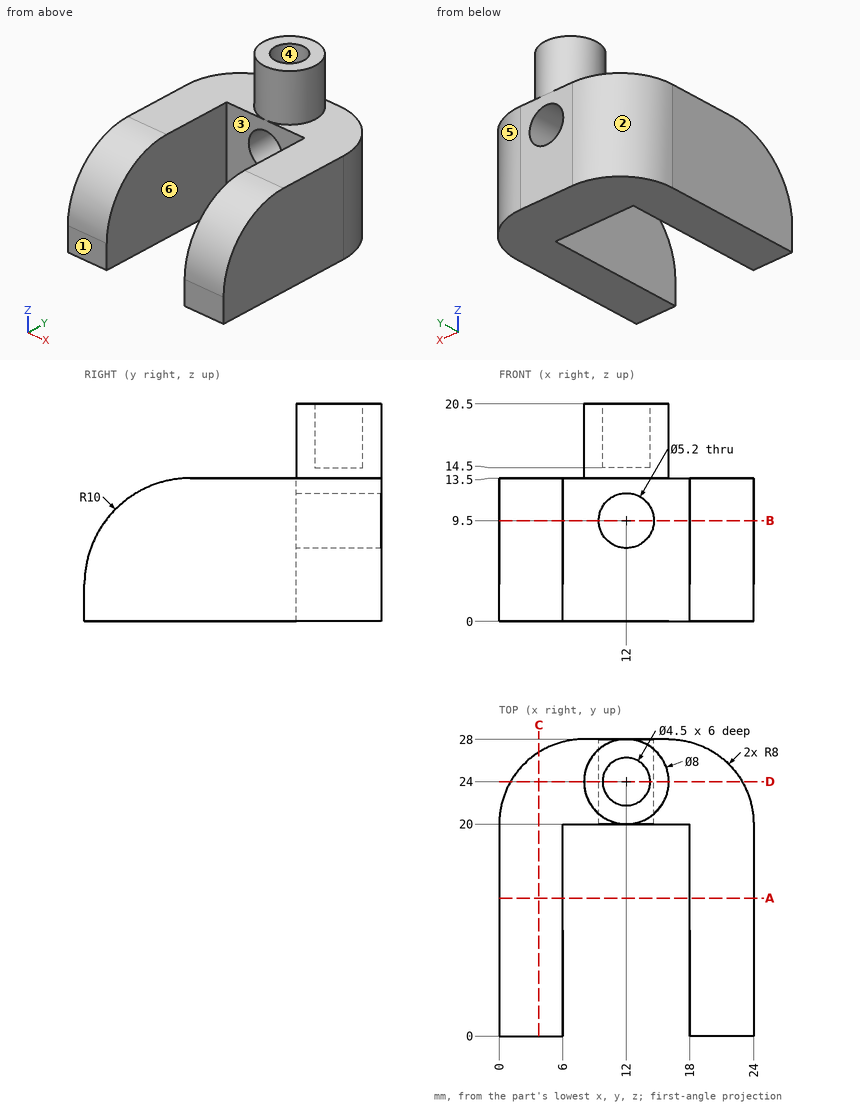
For this review, use the dimensioned drawing (mm, ordinates from the lowest corner) and the shaded views. A direction names the side the tool comes from. Give positions to 0.01 mm unless a question says otherwise; leave off trailing zeros. Order: outer loops, then holes, each group sorted by start corner. A loop starts at its lowest first (then second) coordinate and runs counter-clockwise, first axis right, second up. Notation, with made-up numbers: (37, -14) - (66, -14) arc R23 ccw to (66, -3) - close; hole circle Ø11 at (2, 6). An arc over 180 degrees is marked (long way). Use CSV: the item, a comma, the result in double quotes. Start each with the question number.
Q1. For line 1 (X direction, y = 24, z = 17); line 2 (X direction, y = 18.5, z = 2.75); line 3 (Z direction, x = 12, y = 25), list the stretches that pass through material, from the lowest coordinate up.
Q2. Take a section at A-A (y = 13). State the section outline as (x, z) points, and give its area (3 significant figures).
Q3. For P1, Ø4, axis at x = 12, y = 24, coming from the +Z side; P2, Ø1.5, axis at y = 24, z = 4.5, coming from the -X side; P3, Ø7, axis at x = 12, z = 9.5, coming from the -Y side, all flat-tipped, find the tip position at first contact; note any pin that passes through.
Q4. Draft analysis for pull direction X (two halves, no side actions). For the marked faces 1, 2 and 3, state which applies: pulls with the +X half, pulls with the -X half, needs draft (parallel to the pull), parting line crosses it, or undercut.
Q5. Take a section at D-D (y = 24). State the section outline as (x, z) points.
Q6. Take a section at B-B (z = 9.5). State the section outline as (x, y) points, and give its area (3 significant figures).
Q7. Machinability: for the marked faces 4, 5 and 6, which of the approach directions +Z, -Z, +X, -X, +Y, -Y give a long, thin tool a straight path to every point of the face, cutting with its end or side? Answer none if there is none.
Q8. Take a section at C-C (x = 3.75). State the section outline as (y, z) points.
Calculated:
1,line 1,"x = 8 to 9.75, 14.25 to 16"
1,line 2,"x = 0 to 6, 18 to 24"
1,line 3,"z = 0 to 6.9, 12.1 to 14.5"
2,outline,"(0, 0) - (6, 0) - (6, 13.5) - (0, 13.5) - close; (18, 0) - (24, 0) - (24, 13.5) - (18, 13.5) - close"
2,area,"162 mm²"
3,P1,"stops at z = 14.5"
3,P2,"stops at x = 0.69"
3,P3,"stops at y = 20"
4,face 1,"needs draft"
4,face 2,"pulls with the -X half"
4,face 3,"undercut"
5,outline,"(1.07, 0) - (22.93, 0) - (22.93, 13.5) - (16, 13.5) - (16, 20.5) - (14.25, 20.5) - (14.25, 14.5) - (9.75, 14.5) - (9.75, 20.5) - (8, 20.5) - (8, 13.5) - (1.07, 13.5) - close; hole circle Ø5.2 at (12, 9.5)"
6,outline,"(0, 2) - (6, 2) - (6, 20) - (9.4, 20) - (9.4, 28) - (8, 28) arc R8 ccw to (0, 20) - close; (14.6, 20) - (18, 20) - (18, 2) - (24, 2) - (24, 20) arc R8 ccw to (16, 28) - (14.6, 28) - close"
6,area,"339 mm²"
7,face 4,"+Z"
7,face 5,"+Z, -Z, +X, +Y"
7,face 6,"+Z, -Z, -Y"
8,outline,"(0, 0) - (26.78, 0) - (26.78, 13.5) - (10, 13.5) arc R10 ccw to (0, 3.5) - close"
